Read the model definition and answer for the solid it produces. Units are mm, in the model's axes. Give positions to 0.01 mm unless a question says otherwise; leave off trailing zeros. Loops run counter-clockwise (first coordinate to the right, second up) from the corner with the lowest first, then second, coordinate; pieces in that order, holes last. Notation, with made-up numbers: (9.5, -26.75) - (29.5, -26.75) arc R15 ccw to (29.5, -9.75) - close; hole circle Ø6 at (31, -36). An arc over 180 degrees is marked (long way). Write item = value, one per line.
```python
from build123d import *

# Parameters (mm, degrees)
F0_R     = 40
F1_DEPTH = 10
F4_D     = 10
F5_D     = 15


with BuildPart() as f1:
    # F0 (on Top) → F1 (new body)
    with BuildSketch(Plane.XY):
        Circle(F0_R)
    extrude(amount=F1_DEPTH)

    # F4 (through all)
    with Locations(Plane.XY.offset(10)):
        with Locations((25, 0)):
            Hole(F4_D / 2)

    # F5 (through all)
    with Locations(Plane.XY.offset(10)):
        with Locations((0, 0)):
            Hole(F5_D / 2)


solid = f1.part
```
1) Each of these flat-tipped pins is pushed along its axis until it touches: P1, Ø5, axis at y = 19.5, z = 4, coming from the -X side; P2, Ø2, axis at y = -19.5, z = 5.5, coming from the +X side; P3, Ø1, axis at y = 22.5, z = 2.5, coming from the +X side; P4, Ø8, axis at x = 9, y = -23, coming from the -Z side. Where does it stop, or does it pass through?
Output:
P1 = -36.21
P2 = 35.46
P3 = 33.41
P4 = 0
2) A cutting plane is placed at C-C on z = 6. Determine the outline of the cut face in (x, y), then the cut area to 3 significant figures.
Output:
outline = circle Ø80 at (0, 0); hole circle Ø15 at (0, 0); hole circle Ø10 at (25, 0)
area = 4,770 mm²
3) Find the intervals of material crossed by probe 1 along X at (y, z) = (2.5, 9); probe 2 along X at (y, z) = (1.5, 6.25); probe 3 along Y at (x, z) = (0, 3), in increasing order.
Output:
probe_1 = -39.92 to -7.07, 7.07 to 20.67, 29.33 to 39.92
probe_2 = -39.97 to -7.35, 7.35 to 20.23, 29.77 to 39.97
probe_3 = -40 to -7.5, 7.5 to 40
4) A cutting plane is placed at A-A on y = 0. Determine the outline of the cut face in (x, z), then the cut area to 3 significant figures.
Output:
outline = (-40, 0) - (-7.5, 0) - (-7.5, 10) - (-40, 10) - close; (7.5, 0) - (20, 0) - (20, 10) - (7.5, 10) - close; (30, 0) - (40, 0) - (40, 10) - (30, 10) - close
area = 550 mm²
5) A cutting plane is placed at B-B on x = 25. Determine the outline of the cut face in (y, z).
Output:
outline = (-31.22, 0) - (-5, 0) - (-5, 10) - (-31.22, 10) - close; (5, 0) - (31.22, 0) - (31.22, 10) - (5, 10) - close
6) The mould has two halves that part along Z. Classify faces 1 (the face through (-1, -8, 10)), 2 (the face through (-1, -8, 0)), 3 (the face through (-8.67, -39.05, 4.93)): pulls with the +Z half, pulls with the -Z half, needs draft (parallel to the pull), parting line crosses it, or undercut.
Output:
face_1 = pulls with the +Z half
face_2 = pulls with the -Z half
face_3 = needs draft
7) A cutting plane is placed at D-D on x = 0. Determine the outline of the cut face in (y, z).
Output:
outline = (-40, 0) - (-7.5, 0) - (-7.5, 10) - (-40, 10) - close; (7.5, 0) - (40, 0) - (40, 10) - (7.5, 10) - close
